Part model, mm, in its own coordinate system. A direction names the side the tool comes from. Coordinates: 2 decimals unless noted, no trailing zeros. Order: outer loops, then holes, each group sorted by start corner. A loop starts at its lowest first (then second) coordinate and runs counter-clockwise, first axis right, second up. Notation, with made-up numbers: M 7.5,42.25 L 27.5,42.25 A10 ccw 27.5,53.25 Z; hole C 13.5,77 d9. An arc over 180 degrees is marked long. Write item = value, one per line. Start each with the question number.
Autodesk Inventor part; units mm, degrees
ref_plane "YZ Plane" through (0, 0, 0) normal (1, 0, 0) x (0, 1, 0)
ref_plane "XZ Plane" through (0, 0, 0) normal (0, 1, 0) x (-1, 0, 0)
ref_plane "XY Plane" through (0, 0, 0) normal (0, 0, 1) x (1, 0, 0)
sketch "Náčrt1" plane through (0, 0, 0) normal (0, 0, 1) x (1, 0, 0)
  line L0 (-10, 0) -> (0, 0)
  line L1 (0, 0) -> (0, 20)
  line L2 (0, 20) -> (-1.5, 20)
  line L3 (-1.5, 20) -> (-1.5, 1.5)
  line L4 (-1.5, 1.5) -> (-10, 1.5)
  line L5 (-10, 1.5) -> (-10, 0)
  line L6 (-12, 0) -> (2, 0)
  line L7 (0, 24) -> (0, -4)
  point P0 (0, 0)
  dimension "d0" = 20
  dimension "d1" = 10
  dimension "d2" = 1.5
  dimension "d3" = 1.5
extrude "Vysunutí1" add sketch "Náčrt1" along normal mid plane 25
sketch "Náčrt2" plane through (-10, 1.5, 12.5) normal (0, 1, 0) x (1, 0, 0)
  line L0 (0, 0) -> (0, 25)
  line L1 (8.5, 0) -> (0, 0)
  line L2 (8.5, 25) -> (8.5, 0)
  line L3 (0, 25) -> (8.5, 25)
  point P0 (10, 12.5)
  point P1 (4.25, 20)
  point P2 (4.25, 5)
  point P3 (4.25, 0)
  dimension "d6" = 4.25
  dimension "d7" = 4.25
  dimension "d56" = 15
  dimension "d57" = 5
hole "Díra1" at (-5.75, 1.5, -7.5) at (-5.75, 1.5, 7.5) direction (0, -1, 0) diameter 3.2 end through all
sketch "Náčrt7" plane through (0, 0, 12.5) normal (1, 0, 0) x (0, 0, -1)
  line L0 (25, 20) -> (0, 20)
  line L1 (0, 0) -> (0, 20)
  line L2 (25, 0) -> (0, 0)
  line L3 (25, 20) -> (25, 0)
  point P0 (12.5, 0)
  point P1 (12.5, 10)
  dimension "d58" = 12.5
  dimension "d59" = 10
hole "Díra5" at (0, 10, 0) direction (-1, 0, 0) diameter 8 end through all
sketch "Náčrt8" plane through (0, 0, 12.5) normal (1, 0, 0) x (0, 0, -1)
  circle A0 centre (12.5, 10) radius 4
  line L0 (25, 20) -> (0, 20)
  line L1 (0, 0) -> (0, 20)
  line L2 (25, 0) -> (0, 0)
  line L3 (25, 20) -> (25, 0)
  point P0 (12.5, 0)
  point P1 (22, 8)
  point P2 (3, 8)
  dimension "d67" = 8
  dimension "d68" = 8
  dimension "d69" = 3
  dimension "d70" = 3
hole "Díra6" at (0, 8, -9.5) at (0, 8, 9.5) direction (-1, 0, 0) diameter 2.459 end through all
properties part number "bearing_holder" material "Hliník 6061"
Item 1: Cut at C-C, the plane z = -9.5. Write the cut outline in (x, y).
Item 2: Wall check: line 1 along Z through (x, y) = (-5.75, 0.7); line 2 along Z through (x, y) = (-0.8, 10); line 3 along Y through (x, z) = (-0.4, 0). Give the ranges that are in metal, low to high. Write a range as [from, to].
Item 3: 3-axis set-ups, long thin cutter, end or side, ignore diameter. For faces 1 (the flat face through (-1.5, 13, -3)), 2 (the flat face through (0, 14.3, -0.2)): which of +Z, -Z, +X, -X, +Y, -Y reach the whole face in a straight line?
Item 4: Flat gauge pins, fed straight in: pin 1 (2 mm diameter, centred on y = 6.5, z = -5, fed in from +X); pin 2 (3 mm diameter, centred on x = -6, z = 5, fed in from +Y); pin 3 (5 mm diameter, centred on y = 7, z = 4, fed in from -X). Where does each tip first touch, or does it go through?
Item 5: Pull direction Y, two halves, no side cores. Call faces 3 (the cylindrical face through (-4.19, 0.74, -7.85)), 4 (the cylindrical face through (-0.76, 9.09, 8.93)), 5 (the flat face through (-5, 0, 0)): pulls with the +Y half, pulls with the -Y half, needs draft (parallel to the pull), parting line crosses it, or undercut.
Item 6: Cut at B-B, the plane y = 10. Write the cut outline in (x, z), and give its area (3 significant figures).
Item 7: Cut at A-A, the plane z = 7.5. Write the cut outline in (x, y), and give its area (4 significant figures).
Item 8: Cut at D-D, the plane y = 1. Write the cut outline in (x, z).
Filled sheet:
q1.outline = M -10,0 L 0,0 L 0,6.77 L -1.5,6.77 L -1.5,1.5 L -10,1.5 Z; M -1.5,9.23 L 0,9.23 L 0,20 L -1.5,20 Z
q2.line_1 = [-12.5, -9.1], [-5.9, 5.9], [9.1, 12.5]
q2.line_2 = [-12.5, -4], [4, 12.5]
q2.line_3 = [0, 6], [14, 20]
q3.face_1 = +Z, -Z, -X, +Y
q3.face_2 = +Z, -Z, +X, +Y, -Y
q4.pin_1 = 0
q4.pin_2 = 1.5
q4.pin_3 = -1.5
q5.face_3 = needs draft
q5.face_4 = undercut
q5.face_5 = pulls with the -Y half
q6.outline = M -1.5,-12.5 L 0,-12.5 L 0,-4 L -1.5,-4 Z; M -1.5,4 L 0,4 L 0,12.5 L -1.5,12.5 Z
q6.area = 25.5 mm2
q7.outline = M -10,0 L -7.35,0 L -7.35,1.5 L -10,1.5 Z; M -4.15,0 L 0,0 L 0,20 L -1.5,20 L -1.5,1.5 L -4.15,1.5 Z
q7.area = 37.95 mm2
q8.outline = M -10,-12.5 L 0,-12.5 L 0,12.5 L -10,12.5 Z; hole C -5.75,-7.5 d3.2; hole C -5.75,7.5 d3.2
